from build123d import *

# Parameters (mm, degrees)
SKETCH1_W           = 22.5
SKETCH1_H           = 15
BOSS_EXTRUDE1_DEPTH = 2
SKETCH2_R           = 5
BOSS_EXTRUDE2_DEPTH = 7.5
SKETCH3_W           = 0.269230769
SKETCH3_H           = 3
CUT_EXTRUDE1_DEPTH  = 0.5


with BuildPart() as part:
    # Sketch1 → Boss-Extrude1 (new body)
    with BuildSketch(Plane.XY):
        Rectangle(SKETCH1_W, SKETCH1_H)
    extrude(amount=BOSS_EXTRUDE1_DEPTH)

    # Sketch2 → Boss-Extrude2 (add)
    with BuildSketch(Plane.XY.offset(2)):
        with Locations((3.125, 0)):
            Circle(SKETCH2_R)
    extrude(amount=BOSS_EXTRUDE2_DEPTH)

    # Sketch3 → Cut-Extrude1 (cut)
    with BuildSketch(Plane.XY.offset(2)):
        Polygon((-9.509615385, -1.5), (-9.113581731, 1.5), (-9.075120192, 1.5), (-7.836538462, -0.961538462), (-6.6015625, 1.5), (-6.563100962, 1.5), (-6.163461538, -1.5), (-6.432692308, -1.5), (-6.721153846, 0.656850962), (-7.803485577, -1.5), (-7.864783654, -1.5), (-8.951923077, 0.663461538), (-9.238581731, -1.5), align=None)
        with Locations((-5.413461539, 0)):
            Rectangle(SKETCH3_W, SKETCH3_H)
        with BuildLine():
            Line((-1.740384615, 0.949519231), (-1.975961538, 0.769230769))
            add(Edge.make_bspline(
                [(-1.975961538, 0.769230769), (-1.992766586, 0.789258743), (-2.026150111, 0.829044671), (-2.079857999, 0.884912852), (-2.135830836, 0.937254505), (-2.194047226, 0.986318973), (-2.255555042, 1.030390487), (-2.318864298, 1.071765718), (-2.385034051, 1.10885235), (-2.476535538, 1.153820624), (-2.596233694, 1.2007459), (-2.746914985, 1.240091526), (-2.904210212, 1.265138248), (-3.01152244, 1.26785097), (-3.066105769, 1.269230769)],
                knots=[0, 0, 0, 0, 0.757959112, 1.505699292, 2.245454638, 2.979532153, 3.711538275, 4.438200793, 5.171680507, 5.909471876, 7.393775596, 8.890124382, 10.418191784, 12, 12, 12, 12], degree=3))
            add(Edge.make_bspline(
                [(-3.066105769, 1.269230769), (-3.096177169, 1.268884516), (-3.156040877, 1.268195222), (-3.244882425, 1.259101686), (-3.332065041, 1.246320649), (-3.417532012, 1.227356086), (-3.501174547, 1.203379556), (-3.583539464, 1.174729201), (-3.663434263, 1.139282195), (-3.741964182, 1.100103687), (-3.817203506, 1.055851591), (-3.888393547, 1.007583004), (-3.955274662, 0.955838064), (-4.017899758, 0.90042283), (-4.076332857, 0.841586864), (-4.130150552, 0.778703143), (-4.179166617, 0.711972708), (-4.224352639, 0.642275502), (-4.264820696, 0.569814537), (-4.29870345, 0.49432162), (-4.32870784, 0.417089531), (-4.352450048, 0.337245679), (-4.371242491, 0.25535188), (-4.38420906, 0.171188348), (-4.393199178, 0.084930908), (-4.393885044, 0.026465783), (-4.394230769, -0.003004808)],
                knots=[0, 0, 0, 0, 1.054917814, 2.100044995, 3.131103042, 4.146048494, 5.169673617, 6.183595914, 7.203665975, 8.234915748, 9.262203917, 10.264457458, 11.251630812, 12.227803204, 13.197192746, 14.159520551, 15.12972552, 16.100847026, 17.073214652, 18.039054194, 19.002613845, 19.979014051, 20.95965708, 21.949030935, 22.966165397, 24, 24, 24, 24], degree=3))
            add(Edge.make_bspline(
                [(-4.394230769, -0.003004808), (-4.39314921, -0.047345939), (-4.391025712, -0.134403869), (-4.37212714, -0.261921535), (-4.34340849, -0.384082113), (-4.300366567, -0.500121977), (-4.247293095, -0.611471999), (-4.180229714, -0.716248159), (-4.102558396, -0.816033785), (-4.013180323, -0.908470598), (-3.915118195, -0.992910934), (-3.809905699, -1.067268575), (-3.697804881, -1.12925276), (-3.580053483, -1.180832143), (-3.455745386, -1.220480766), (-3.325104127, -1.248392872), (-3.188413845, -1.266600456), (-3.095011502, -1.268343617), (-3.047475962, -1.269230769)],
                knots=[0, 0, 0, 0, 1.029171465, 2.020641659, 2.987623507, 3.938342917, 4.889210282, 5.84687017, 6.821220943, 7.821438502, 8.827599549, 9.822697543, 10.807740252, 11.797342354, 12.80366471, 13.83203677, 14.896651826, 16, 16, 16, 16], degree=3))
            add(Edge.make_bspline(
                [(-3.047475962, -1.269230769), (-2.995102228, -1.267783244), (-2.892018192, -1.264934167), (-2.740845598, -1.240797668), (-2.596129227, -1.20166231), (-2.457861296, -1.146892662), (-2.326431599, -1.075693844), (-2.201634462, -0.989381378), (-2.083364544, -0.887134235), (-2.012246302, -0.809062982), (-1.975961538, -0.769230769)],
                knots=[0, 0, 0, 0, 1.028121516, 2.023589091, 2.998037872, 3.967518031, 4.937445131, 5.927275754, 6.942489185, 8, 8, 8, 8], degree=3))
            Line((-1.975961538, -0.769230769), (-1.740384615, -0.947716346))
            add(Edge.make_bspline(
                [(-1.740384615, -0.947716346), (-1.759342995, -0.972177876), (-1.797168946, -1.020983767), (-1.858418674, -1.08978809), (-1.922942072, -1.154505835), (-1.991218395, -1.214615224), (-2.062462216, -1.271319052), (-2.13795277, -1.323006336), (-2.216697655, -1.370398523), (-2.298430065, -1.413793029), (-2.383063162, -1.452293527), (-2.470495535, -1.485253899), (-2.560350314, -1.513646662), (-2.652631607, -1.537005464), (-2.747530827, -1.555237822), (-2.844705519, -1.567426115), (-2.944365412, -1.575776327), (-3.011600916, -1.576537398), (-3.045673077, -1.576923077)],
                knots=[0, 0, 0, 0, 0.986787822, 1.968848986, 2.935600012, 3.899624008, 4.868462664, 5.837806735, 6.815139263, 7.798259679, 8.787526145, 9.778297419, 10.776456485, 11.791383307, 12.812564526, 13.85620153, 14.913611965, 16, 16, 16, 16], degree=3))
            add(Edge.make_bspline(
                [(-3.045673077, -1.576923077), (-3.077939077, -1.576698512), (-3.141741097, -1.576254462), (-3.235940027, -1.569061176), (-3.327645382, -1.559247116), (-3.416595062, -1.544469861), (-3.503274469, -1.527031855), (-3.586897827, -1.503656492), (-3.668288007, -1.477471492), (-3.747118014, -1.446695789), (-3.823454899, -1.411967633), (-3.897052452, -1.372717725), (-3.967876822, -1.329276127), (-4.036624326, -1.282600404), (-4.102279398, -1.231191288), (-4.165410991, -1.175762744), (-4.226373113, -1.116501592), (-4.2640897, -1.07376886), (-4.283052885, -1.052283654)],
                knots=[0, 0, 0, 0, 1.114604814, 2.203992996, 3.262667896, 4.300477797, 5.318619304, 6.316056647, 7.298880507, 8.271930387, 9.238335007, 10.195173496, 11.151986948, 12.108099108, 13.064862484, 14.031167946, 15.010108607, 16, 16, 16, 16], degree=3))
            add(Edge.make_bspline(
                [(-4.283052885, -1.052283654), (-4.313426293, -1.014962635), (-4.373806416, -0.940771169), (-4.451057002, -0.820526042), (-4.517183478, -0.694981863), (-4.570648553, -0.563479067), (-4.612445181, -0.426312735), (-4.641400492, -0.283413723), (-4.660216153, -0.134915486), (-4.662367829, -0.033912525), (-4.663461538, 0.017427885)],
                knots=[0, 0, 0, 0, 0.994628077, 1.977248131, 2.950237994, 3.925870899, 4.908910175, 5.911660606, 6.938484602, 8, 8, 8, 8], degree=3))
            add(Edge.make_bspline(
                [(-4.663461538, 0.017427885), (-4.662128515, 0.071389702), (-4.659505876, 0.177556209), (-4.637223765, 0.333362454), (-4.601379083, 0.482635082), (-4.550467464, 0.625095434), (-4.48592002, 0.761492818), (-4.406182923, 0.890785279), (-4.312182515, 1.013799679), (-4.204656028, 1.128669465), (-4.08674117, 1.233703196), (-3.960467901, 1.326108514), (-3.826083375, 1.403009242), (-3.685068073, 1.467291667), (-3.53636606, 1.516701206), (-3.380294601, 1.551289652), (-3.21714696, 1.572818609), (-3.105836309, 1.575540216), (-3.049278846, 1.576923077)],
                knots=[0, 0, 0, 0, 1.032925535, 2.032216505, 3.007276963, 3.968222605, 4.92396291, 5.891752235, 6.871517503, 7.883894988, 8.900124299, 9.891468569, 10.874487609, 11.85992873, 12.854644235, 13.869047385, 14.917252991, 16, 16, 16, 16], degree=3))
            add(Edge.make_bspline(
                [(-3.049278846, 1.576923077), (-3.014809299, 1.576509816), (-2.946580301, 1.575691806), (-2.845649456, 1.567715113), (-2.747384604, 1.554417736), (-2.651718048, 1.536318248), (-2.558184377, 1.51385483), (-2.467498457, 1.484591717), (-2.379128154, 1.451131833), (-2.293630804, 1.412596005), (-2.211416618, 1.369338798), (-2.132511202, 1.321839692), (-2.057541323, 1.270157573), (-1.985979453, 1.214731994), (-1.919022701, 1.154390372), (-1.854770005, 1.090792432), (-1.795403366, 1.022106297), (-1.758757771, 0.973759211), (-1.740384615, 0.949519231)],
                knots=[0, 0, 0, 0, 1.096760587, 2.17092713, 3.219439832, 4.250915756, 5.268269357, 6.278326846, 7.281116186, 8.274029601, 9.260640565, 10.235837813, 11.203064059, 12.156899882, 13.114053108, 14.069676657, 15.032185724, 16, 16, 16, 16], degree=3))
        make_face()
    extrude(amount=-CUT_EXTRUDE1_DEPTH, mode=Mode.SUBTRACT)


solid = part.part
The listing builds one solid part. Answer for the finished solid, in the listing's coordinates (mm). A direction names the side the tool comes from. Round coordinates to 2 decimals unless told otherwise and drop trailing zeros. Write each loop counter-clockwise with the first axis right and the second up, starting at its lowest first coordinate (ties: lowest second). Pieces come first, ordered by that corner, then holes. Notation, with made-up numbers: M 29,69.25 L 70,69.25 A23 cw 70,96.25 Z; hole C -32.5,-6 d9. An arc over 180 degrees is marked long. Write each question's results on one line, items separated by ' | '. Start each with the question number.
Item 1: For faces 4 (the face through (-7.23, 0.25, 1.75)), 5 (the face through (3, 0, 9.5)), determine the directions among +Z, -Z, +X, -X, +Y, -Y from which every point of the face is accessible in a straight line to the end or side of a thin tool.
Item 2: A cutting plane is placed at C-C on x = 8.5. Write down the section's boundary in (y, z).
Item 3: Straight lines are drawn through the part: L1, parallel to Z at x = -3, y = -2.5; L2, parallel to X at y = 0, z = 6.75 (3 decimals); L3, parallel to Y at x = -1.25, z = 3.5. For each, find the intervals that lie inside material, in ascending order. Write a range as [from, to].
Item 4: A cutting plane is placed at B-B on z = 6. Write down the section's boundary in (x, y) (3 decimals), and give its area (3 significant figures).
Item 5: A cutting plane is placed at D-D on y = 4.5. Write down the section's boundary in (x, z).
Item 6: Flat-ended cylindrical pins translate along their axes: pin 1 Ø3 at (y, z) = (1.5, 4) entering from -X (3 decimals); pin 2 Ø2.5 at (x, y) = (-3.5, 0.5) entering from +Z. Find the tip coordinate at first contact, or state that the pin passes through.
Item 7: For a pull along X with two mould halves and no side action, classify faces 1 (the face through (0, 7.5, 1)), 2 (the face through (-8.464, 0.286, 1.754)), 3 (the face through (11.25, 0, 1)) as pulls with the +X half, pulls with the -X half, needs draft (parallel to the pull), parting line crosses it, or undercut.
Item 8: A cutting plane is placed at A-A on y = 2.25. Write down the section's boundary in (x, z), and give its area (3 significant figures).
Check sheet entries:
1) face 4: +Z | face 5: +Z, +X, -X, +Y, -Y
2) outline: M -7.5,0 L 7.5,0 L 7.5,2 L -7.5,2 Z
3) L1: [0, 2] | L2: [-1.875, 8.125] | L3: [-2.42, 2.42]
4) outline: C 3.125,0 d10 | area: 78.5 mm²
5) outline: M -11.25,0 L 11.25,0 L 11.25,2 L 5.3,2 L 5.3,9.5 L 0.95,9.5 L 0.95,2 L -11.25,2 Z
6) pin 1: x = -1.875 | pin 2: z = 2
7) face 1: needs draft | face 2: undercut | face 3: pulls with the +X half
8) outline: M -11.25,0 L 11.25,0 L 11.25,2 L 7.59,2 L 7.59,9.5 L -1.34,9.5 L -1.34,2 L -11.25,2 Z | area: 112 mm²
